Geometry check sheet. Reference: the model listing, model coordinates, mm. Face numbers are marked on the shaded views. A direction names the side the tool comes from. Round coordinates to 2 decimals unless told otherwise and drop trailing zeros. Write each loop counter-clockwise with the first axis right and the second up, starting at its lowest first coordinate (ties: lowest second). Pieces come first, ordered by that corner, then holes.
Item 1: Depth check by flat-ended pin: P1, Ø2.5, axis at x = -12, z = 0.5, coming from the -Y side; P2, Ø2, axis at y = 7, z = -3.5, coming from the -X side; P3, Ø6, axis at y = 7, z = -0.5, coming from the +X side; P4, Ø10, axis at x = -14.5, y = 3.5, coming from the +Z side. Enter the tip coordinate at first touch or a pass-through.
Item 2: Draft check along X on the marked faces 1, 2, 3 and 4. Enter one of: pulls with the +X half, pulls with the -X half, needs draft (parallel to the pull), parting line crosses it, or undercut.
Item 3: Cross-section at C-C (y = 12). Enter the section's corners in (x, z).
Item 4: Cross-section at D-D (z = 3.5). Enter the section's corners in (x, y).
Item 5: Scan lines: probe 1 along X at (y, z) = (12, 2); probe 2 along Z at (x, y) = (-5, 11); probe 3 along Y at (x, z) = (-12.5, 3.75). Record each from-to range of solid material in increasing order.
Item 6: Cross-section at A-A (y = 1.25). Enter the section's corners in (x, z), then the cut area to 3 significant figures.
Item 7: Cross-section at B-B (x = 0). Enter the section's corners in (y, z).
Item 8: Access from +Z, -Z, +X, -X, +Y, -Y to the whole of each face (thin tool, end or side, straight path). Record for the marked faces 5, 6, 7 and 8.
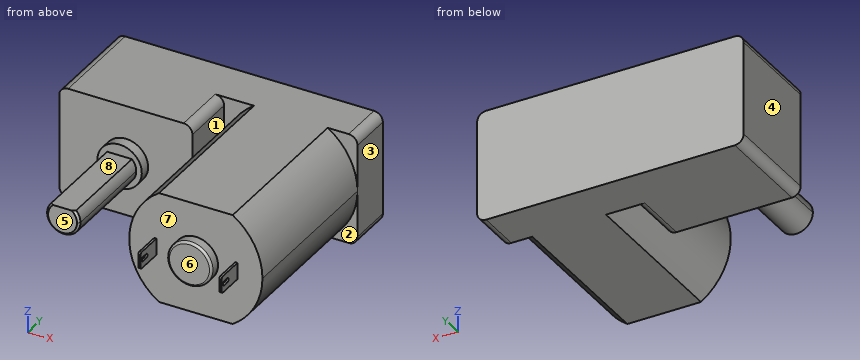
from build123d import *

# Parameters (mm, degrees)
EXTRUDE_1_DEPTH     = 15
SKETCH_2_R          = 2
EXTRUDE_2_DEPTH     = 1
SKETCH_4_W          = 24
SKETCH_4_H          = 10
EXTRUDE_3_DEPTH     = 4
SKETCH_5_W          = 11.99
SKETCH_5_H          = 10
EXTRUDE_6_DEPTH     = 5
EXTRUDE_7_DEPTH     = 10
SKETCH_7_R          = 2
EXTRUDE_8_DEPTH     = 1
SKETCH_8_W          = 0.2
SKETCH_8_H          = 1.5
EXTRUDE_9_DEPTH     = 2.5
CUT_EXTRUDE_1_DEPTH = 9.5
FILLET_1_R          = 0.2
FILLET_2_R          = 0.2
FILLET_3_R          = 0.8
CHAMFER_1_SIZE      = 0.2


with BuildPart() as part:
    # 草图1 → 凸台-拉伸1 (new body)
    with BuildSketch(Plane(origin=(0, 0, 0), x_dir=(1, 0, 0), z_dir=(0, 1, 0))):
        with BuildLine():
            Line((3.31662479, 5), (-3.31662479, 5))
            ThreePointArc((-3.31662479, 5), (-6, 0), (-3.31662479, -5))
            Line((-3.31662479, -5), (3.31662479, -5))
            ThreePointArc((3.31662479, -5), (5.286764074, -2.837274331), (6, 0))
            ThreePointArc((6, 0), (5.286764074, 2.837274331), (3.31662479, 5))
        make_face()
    extrude(amount=EXTRUDE_1_DEPTH)

    # 草图2 → 凸台-拉伸2 (add)
    with BuildSketch(Plane.XZ):
        with Locations(Location((0, 0, 0), (0, 0, 270))):
            Circle(SKETCH_2_R)
    extrude(amount=EXTRUDE_2_DEPTH)

    # 草图4 → 凸台-拉伸3 (add)
    with BuildSketch(Plane(origin=(0, 15, 0), x_dir=(1, 0, 0), z_dir=(0, 1, 0))):
        with Locations((-6, 0)):
            Rectangle(SKETCH_4_W, SKETCH_4_H)
    extrude(amount=EXTRUDE_3_DEPTH)

    # 草图5 → 凸台-拉伸6 (add)
    with BuildSketch(Plane.XZ.offset(-15)):
        with Locations((-12.005, 0)):
            Rectangle(SKETCH_5_W, SKETCH_5_H)
    extrude(amount=EXTRUDE_6_DEPTH)

    # 草图6 → 凸台-拉伸7 (add)
    with BuildSketch(Plane.XZ.offset(-10)):
        with BuildLine():
            ThreePointArc((-13.118033989, 1), (-13.401258538, 0.535233135), (-13.5, 0))
            Line((-13.5, 0), (-10.5, 0))
            ThreePointArc((-10.5, 0), (-10.598741462, 0.535233135), (-10.881966011, 1))
            Line((-10.881966011, 1), (-13.118033989, 1))
        make_face()
        with BuildLine():
            Line((-10.5, 0), (-13.5, 0))
            ThreePointArc((-13.5, 0), (-12, -1.5), (-10.5, 0))
        make_face()
    extrude(amount=EXTRUDE_7_DEPTH)

    # 草图7 → 凸台-拉伸8 (add)
    with BuildSketch(Plane.XZ.offset(-10)):
        with Locations(Location((-12, 0, 0), (0, 0, 270))):
            Circle(SKETCH_7_R)
    extrude(amount=EXTRUDE_8_DEPTH)

    # 草图8 → 凸台-拉伸9 (add)
    with BuildSketch(Plane.XZ):
        with Locations((-3.65, 0)):
            Rectangle(SKETCH_8_W, SKETCH_8_H)
        with Locations((3.65, 0)):
            Rectangle(SKETCH_8_W, SKETCH_8_H)
    extrude(amount=EXTRUDE_9_DEPTH)

    # 草图9 → 切除-拉伸1 (cut)
    with BuildSketch(Plane(origin=(3.75, 0, 0), x_dir=(0, 0, -1), z_dir=(1, 0, 0))):
        with BuildLine():
            Line((-0.2, -2.1), (-0.2, -1.6))
            ThreePointArc((-0.2, -1.6), (0, -1.4), (0.2, -1.6))
            Line((0.2, -1.6), (0.2, -2.1))
            ThreePointArc((0.2, -2.1), (0, -2.3), (-0.2, -2.1))
        make_face()
    extrude(amount=-CUT_EXTRUDE_1_DEPTH, mode=Mode.SUBTRACT)

    # 圆角1
    fillet_1_edges = [part.edges().sort_by_distance(p)[0] for p in [
        (-3.65, -2.5, 0.75),
        (-3.65, -2.5, -0.75),
        (3.65, -2.5, 0.75),
        (3.65, -2.5, -0.75),
    ]]
    fillet(fillet_1_edges, radius=FILLET_1_R)

    # 圆角2
    fillet_2_edges = [part.edges().sort_by_distance(p)[0] for p in [
        (0, -1, 2),
    ]]
    fillet(fillet_2_edges, radius=FILLET_2_R)

    # 圆角3
    fillet_3_edges = [part.edges().sort_by_distance(p)[0] for p in [
        (-18, 14.5, 5),
        (6, 17, 5),
        (6, 17, -5),
        (-18, 14.5, -5),
        (-6.01, 12.5, -5),
        (-6.01, 12.5, 5),
    ]]
    fillet(fillet_3_edges, radius=FILLET_3_R)

    # 倒角1
    chamfer_1_edges = [part.edges().sort_by_distance(p)[0] for p in [
        (-12.535233135, 0, -1.401258538),
    ]]
    chamfer(chamfer_1_edges, length=CHAMFER_1_SIZE)


solid = part.part
Resolved:
1. P1: stops at y = 0
1. P2: stops at x = -5.45
1. P3: stops at x = 6
1. P4: stops at z = 1
2. face 1: undercut
2. face 2: needs draft
2. face 3: pulls with the +X half
2. face 4: pulls with the -X half
3. outline: (-18, -4.2) arc R0.8 ccw to (-17.2, -5) - (-6.81, -5) arc R0.8 ccw to (-6.01, -4.2) - (-6.01, 4.2) arc R0.8 ccw to (-6.81, 5) - (-17.2, 5) arc R0.8 ccw to (-18, 4.2) - close; (-3.32, -5) - (3.32, -5) arc R6 ccw to (3.32, 5) - (-3.32, 5) arc R6 ccw to start
4. outline: (-18, 10) - (-6.01, 10) - (-6.01, 15) - (-4.87, 15) - (-4.87, 0) - (4.87, 0) - (4.87, 15) - (6, 15) - (6, 19) - (-18, 19) - close
5. probe 1: x = -18 to -6.01, -5.66 to 5.66
5. probe 2: z = -3.32 to 3.32
5. probe 3: y = 10 to 19
6. outline: (-13.12, 1) arc R1.5 ccw (long way) to (-10.88, 1) - close; (-3.32, -5) - (3.32, -5) arc R6 ccw to (3.32, 5) - (-3.32, 5) arc R6 ccw to start
6. area: 110 mm2
7. outline: (-1, -1.8) arc R0.2 ccw to (-0.8, -2) - (0, -2) - (0, -5) - (19, -5) - (19, 5) - (0, 5) - (0, 2) - (-0.8, 2) arc R0.2 ccw to (-1, 1.8) - close
8. face 5: +Z, -Z, -X, -Y
8. face 6: +Z, -Z, -Y
8. face 7: -Y
8. face 8: +Z, -X, -Y
